Geometry check sheet. Reference: the model listing, model coordinates, mm. A direction names the side the tool comes from. Give positions to 0.01 mm unless a question says otherwise; leave off trailing zeros. Write each loop counter-clockwise with the first axis right and the second up, starting at its lowest first coordinate (ties: lowest second). Pieces come first, ordered by that corner, then holes. Notation, with made-up numbers: (32, 45) -> (59, 45) arc R16 ccw to (59, 76) -> close; hole circle Ø5 at (-23.75, 26). An arc over 180 degrees is marked (long way). Write item = value, one per line. Start each with the question number.
1. Cross-section at A-A, the plane y = 9. Record the cut outline in (x, z).
2. Mould release check, pull along Y, two halves, no side actions. Record for faces 6 (the flat face through (19, 27, 10)), 7 (the flat face through (14, 27.5, 4)), 8 (the flat face through (65.5, 0, 5)), 9 (the flat face through (-37, 13.5, 9)): pulls with the +Y half, pulls with the -Y half, needs draft (parallel to the pull), parting line crosses it, or undercut.
3. Thickness scan on line 1 along X through (y, z) = (5, 7.25); line 2 along X through (y, z) = (20.5, 2.5); line 3 along Y through (x, z) = (59, 7). Record the ranges inside material, lowest first.
4. Cross-section at D-D, the plane y = 18. Record the cut outline in (x, z).
5. Depth check by flat-ended pin: P1, Ø1, axis at x = -36.5, z = 9.5, coming from the -Y side; P2, Ø10, axis at x = 8, y = 10, coming from the +Z side; P3, Ø0.6, axis at x = -36, y = 20, coming from the +Z side. Enter the tip coordinate at first touch or a pass-through.
6. Cross-section at B-B, the plane x = -14. Record the cut outline in (y, z), plus the area to 3 significant figures.
7. Cross-section at C-C, the plane z = 5. Record the cut outline in (x, y), plus the area to 3 significant figures.
8. Set-up check for faces 1 (the flat face through (35.5, 0, 6)), 2 (the flat face through (-37.5, 6, 3)), 3 (the flat face through (-36, -18, 4)), 4 (the cylindrical face through (36.31, -23.83, 4.07)), 5 (the flat face through (-37, 23.5, 9)): record each of +Z, -Z, +X, -X, +Y, -Y from which the full face is reachable in a straight line by a thin tool's end or side.
Autodesk Fusion 360 part; units mm, degrees
sketch "Sketch1" plane through (0, 0, 0) normal (0, 0, 1) x (1, 0, 0)
  line L0 (35.5, -25.5) -> (-35.5, -25.5)
  line L1 (-35.5, -25.5) -> (-35.5, 25.5)
  line L2 (-35.5, 25.5) -> (35.5, 25.5)
  line L3 (35.5, 25.5) -> (35.5, -25.5)
  line L4 (35.5, -25.5) -> (-35.5, 25.5) construction
  line L5 (-35.5, -25.5) -> (35.5, 25.5) construction
  line L6 (34.5, -24.5) -> (-34.5, -24.5)
  line L7 (-34.5, -24.5) -> (-34.5, 24.5)
  line L8 (-34.5, 24.5) -> (34.5, 24.5)
  line L9 (34.5, 24.5) -> (34.5, -24.5)
  line L10 (-37.5, -27.5) -> (-37.5, 27.5)
  line L11 (-37.5, 27.5) -> (37.5, 27.5)
  line L12 (37.5, 27.5) -> (37.5, -27.5)
  line L13 (37.5, -27.5) -> (-37.5, -27.5)
  line L14 (37.5, -27.5) -> (67.5, -27.5)
  line L15 (67.5, -27.5) -> (67.5, 27.5)
  line L16 (67.5, 27.5) -> (37.5, 27.5)
  line L17 (37.5, 27.5) -> (37.5, -27.5)
  line L18 (37.5, -25.5) -> (65.5, -25.5)
  line L19 (65.5, -25.5) -> (65.5, 25.5)
  line L20 (65.5, 25.5) -> (37.5, 25.5)
  dimension "d1" = 71
  dimension "d2" = 51
  dimension "d3" = 1
  dimension "d4" = -2
  dimension "d5" = 30
  dimension "d6" = 55
  dimension "d7" = -2
extrude "Extrude1" add sketch "Sketch1" along normal blind 10 contours L10 L11 L12 L13 L17 | L12 L14 L15 L16 L17 L18 L19 L20
extrude "Extrude2" add sketch "Sketch1" against normal blind 1 contours L0 L1 L2 L3 | L6 L7 L8 L9 | L10 L11 L12 L13 L17 | L12 L14 L15 L16 L17 L18 L19 L20 | L12 L17 L18 L19 L20
extrude "Extrude3" add sketch "Sketch1" along normal blind 3 contours L0 L1 L2 L3
hole "Hole1" at (37.5, -21.7224, 5.415) direction (-1, 0, 0) diameter 5 depth 5 tip angle 118
sketch "Sketch2" plane through (0, 0, 10) normal (0, 0, 1) x (-1, 0, 0)
  line L0 (35.5, -25.5) -> (-35.5, -25.5)
  line L1 (-35.5, -25.5) -> (-35.5, 25.5)
  line L2 (-35.5, 25.5) -> (35.5, 25.5)
  line L3 (35.5, 25.5) -> (35.5, -25.5)
  line L4 (-37.5, -25.5) -> (-65.5, -25.5)
  line L5 (-65.5, -25.5) -> (-65.5, 25.5)
  line L6 (-65.5, 25.5) -> (-37.5, 25.5)
  line L7 (-37.5, 25.5) -> (-37.5, -25.5)
  line L8 (37.5, 27.5) -> (-67.5, 27.5)
  line L9 (-67.5, 27.5) -> (-67.5, -27.5)
  line L10 (-67.5, -27.5) -> (37.5, -27.5)
  line L11 (37.5, -27.5) -> (37.5, 27.5)
  line L12 (37.5, 0) -> (23.5, 0)
  line L13 (23.5, 0) -> (23.5, 27.5)
  line L14 (23.5, 27.5) -> (37.5, 27.5)
  line L15 (37.5, 27.5) -> (37.5, 0)
  dimension "d17" = 14
extrude "Extrude4" cut sketch "Sketch2" against normal blind 6 contours L2 L3 L8 L11 L12 L13 L14 L15
sketch "Sketch3" plane through (0, -27.5, 0) normal (0, -1, 0) x (1, 0, 0)
  line L0 (-23.5, 4) -> (-37.5, 4)
  line L1 (-37.5, 4) -> (-37.5, -1)
  line L2 (-37.5, -1) -> (67.5, -1)
  line L3 (67.5, -1) -> (67.5, 10)
  line L4 (67.5, 10) -> (-23.5, 10)
  line L5 (-23.5, 10) -> (-23.5, 4)
  line L6 (-23.5, 4) -> (0.8403, 28.3403)
  line L7 (-23.5, 4) -> (10.9224, 4) construction
  line L8 (-17.5, 10) -> (-17.5, 4)
  line L9 (-23.5, 4) -> (-17.5, 4)
  dimension "d23" = 45
extrude "Extrude5" cut sketch "Sketch3" against normal blind 8 contours L4 L5 L6
sketch "Sketch4" plane through (-37.5, 0, 0) normal (-1, 0, 0) x (0, -1, 0)
  line L0 (27.5, 4) -> (0, 4)
  line L1 (0, 4) -> (0, 10)
  line L2 (0, 10) -> (-27.5, 10)
  line L3 (-27.5, 10) -> (-27.5, -1)
  line L4 (-27.5, -1) -> (27.5, -1)
  line L5 (27.5, -1) -> (27.5, 4)
  line L6 (-27.5, 10) -> (-23.5, 10)
  line L7 (-23.5, 10) -> (-13.5, 10)
  line L8 (0, 4) -> (-6, 10)
  line L9 (0, 4) -> (8.4853, 4) construction
  line L10 (0, 4) -> (-27.5, 4)
  line L11 (-6, 10) -> (-6, 4)
  line L12 (-13.5, 10) -> (-13.5, 8)
  line L13 (-23.5, 10) -> (-23.5, 8)
  line L14 (-23.5, 8) -> (-13.5, 8)
  dimension "d26" = 4
  dimension "d27" = 10
  dimension "d28" = 135
  dimension "d29" = 2
extrude "Extrude6" cut sketch "Sketch4" against normal blind 5.5 contours L1 L2 L8 | L2 L7 L12 L13 L14
Answers:
q1.outline = (-37.5, -1) -> (67.5, -1) -> (67.5, 10) -> (65.5, 10) -> (65.5, 0) -> (37.5, 0) -> (37.5, 10) -> (35.5, 10) -> (35.5, 3) -> (34.5, 3) -> (34.5, 0) -> (-34.5, 0) -> (-34.5, 3) -> (-35.5, 3) -> (-35.5, 10) -> (-37.5, 10) -> close
q2.face_6 = needs draft
q2.face_7 = pulls with the +Y half
q2.face_8 = undercut
q2.face_9 = undercut
q3.line_1 = -37.5 to -35.5, 35.5 to 37.5, 65.5 to 67.5
q3.line_2 = -37.5 to -34.5, 34.5 to 37.5, 65.5 to 67.5
q3.line_3 = -27.5 to -25.5, 25.5 to 27.5
q4.outline = (-37.5, -1) -> (67.5, -1) -> (67.5, 10) -> (65.5, 10) -> (65.5, 0) -> (37.5, 0) -> (37.5, 10) -> (35.5, 10) -> (35.5, 3) -> (34.5, 3) -> (34.5, 0) -> (-34.5, 0) -> (-34.5, 3) -> (-35.5, 3) -> (-35.5, 8) -> (-37.5, 8) -> close
q5.P1 = 5
q5.P2 = 0
q5.P3 = 8
q6.outline = (-27.5, -1) -> (27.5, -1) -> (27.5, 10) -> (25.5, 10) -> (25.5, 3) -> (24.5, 3) -> (24.5, 0) -> (-24.5, 0) -> (-24.5, 3) -> (-25.5, 3) -> (-25.5, 10) -> (-27.5, 10) -> close
q6.area = 101 mm^2
q7.outline = (-37.5, 1) -> (-35.5, 1) -> (-35.5, 25.5) -> (35.5, 25.5) -> (35.5, -19.26) -> (37.5, -19.26) -> (37.5, 25.5) -> (65.5, 25.5) -> (65.5, -25.5) -> (37.5, -25.5) -> (37.5, -24.19) -> (35.5, -24.19) -> (35.5, -25.5) -> (-22.5, -25.5) -> (-22.5, -27.5) -> (67.5, -27.5) -> (67.5, 27.5) -> (-37.5, 27.5) -> close
q7.area = 633 mm^2
q8.face_1 = +Z
q8.face_2 = +Z, -Z, -X, +Y, -Y
q8.face_3 = +Z, -X, -Y
q8.face_4 = none
q8.face_5 = +Z, -X
